For this review, take the finished solid that the model builds, in its own axes (mm). A direction names the side the tool comes from. Round coordinates to 2 decimals unless told otherwise and drop trailing zeros. Write each loop counter-clockwise with the first axis right and the second up, starting at its lowest first coordinate (ties: lowest second). Pieces come first, ordered by that corner, then holes. Notation, with made-up numbers: (75.5, 46) -> (131.5, 46) arc R10 ccw to (131.5, 63) -> close; hole circle Ø7 at (-38.5, 22.5). An arc over 180 degrees is marked (long way). Write each question's results on one line, items separated by ' | '. Start each with the question number.
Item 1: Add section D-D (x = -91). State the section outline as (y, z) points.
Item 2: Add section A-A (y = 0). State the section outline as (x, z) points.
Item 3: Add section C-C (z = 278). State the section outline as (x, y) points, plus the area to 3 significant figures.
Item 4: Tool access review of faces 5 (the flat face through (-1, 111, -45.487)), 6 (the flat face through (2, -54, 0)), 7 (the cylindrical face through (124.88, 5.5, -57.89)): name each direction out of +Z, -Z, +X, -X, +Y, -Y from which nothing blocks a thin tool from reaching the whole face with its end or side.
Item 5: To check wall thickness, follow line 1 along Z through (x, y) = (-100, -70.5); line 2 along Z through (x, y) = (-71, -68.5); line 3 along Y through (x, z) = (32, 986). State the ranges of each line that lie inside material, in increasing order.
Item 6: The part is to be moulded in two halves that separate along Z. For faces 1 (the flat face through (-1, 111, -25.487)), 2 (the flat face through (-1, 1, 1200)), 3 (the cylindrical face through (47.69, 15.02, 591.6)), 4 (the flat face through (2, 2, -70.65)), say which applies: +Z half, -Z half, draft (parallel to the pull), parting line (faces both ways), or undercut.
Item 7: Clearance check with flat-ended pins moving along their axes: pin 1 (5 mm diameter, centred on x = -42, z = 1028, fed in from -Y); pin 2 (6 mm diameter, centred on x = 32, z = 545.5, fed in from +Y); pin 3 (1 mm diameter, centred on y = 17.5, z = 1015.5, fed in from -X). State where each tip first meets the part, or that it passes through.
from build123d import *

# Parameters (mm, degrees)
SKETCH1_R           = 50
BOSS_EXTRUDE1_DEPTH = 1200
SKETCH2_R           = 125
BOSS_EXTRUDE2_DEPTH = 70.65
SKETCH5_W           = 15
SKETCH5_H           = 20


with BuildPart() as part:
    # Sketch1 → Boss-Extrude1 (new body)
    with BuildSketch(Plane.XY):
        Circle(SKETCH1_R)
    extrude(amount=BOSS_EXTRUDE1_DEPTH)

    # Sketch2 → Boss-Extrude2 (add)
    with BuildSketch(Plane(origin=(0, 0, 0), x_dir=(-1, 0, 0), z_dir=(0, 0, -1))):
        Circle(SKETCH2_R)
    extrude(amount=BOSS_EXTRUDE2_DEPTH)

    # Sketch5 → Cut-Revolve1 (revolve, cut)
    with BuildSketch(Plane(origin=(0, 0, 0), x_dir=(1, 0, 0), z_dir=(0, 1, 0)), mode=Mode.PRIVATE) as cut_revolve1_sk:
        with Locations((-117.5, 35.486594565)):
            Rectangle(SKETCH5_W, SKETCH5_H)
    revolve(cut_revolve1_sk.sketch.rotate(Axis((0, 0, 1200), (0, 0, -1)), 180), axis=Axis((0, 0, 1200), (0, 0, -1)), mode=Mode.SUBTRACT)


solid = part.part
Responses:
1) outline: (-85.7, -70.65) -> (85.7, -70.65) -> (85.7, -45.49) -> (61.8, -45.49) -> (61.8, -25.49) -> (85.7, -25.49) -> (85.7, 0) -> (-85.7, 0) -> (-85.7, -25.49) -> (-61.8, -25.49) -> (-61.8, -45.49) -> (-85.7, -45.49) -> close
2) outline: (-125, -70.65) -> (125, -70.65) -> (125, -45.49) -> (110, -45.49) -> (110, -25.49) -> (125, -25.49) -> (125, 0) -> (50, 0) -> (50, 1200) -> (-50, 1200) -> (-50, 0) -> (-125, 0) -> (-125, -25.49) -> (-110, -25.49) -> (-110, -45.49) -> (-125, -45.49) -> close
3) outline: circle Ø100 at (0, 0) | area: 7,850 mm^2
4) face 5: none | face 6: +Z | face 7: +Z, -Z
5) line 1: z = -70.65 to -45.49, -25.49 to 0 | line 2: z = -70.65 to 0 | line 3: y = -38.42 to 38.42
6) face 1: undercut | face 2: +Z half | face 3: draft | face 4: -Z half
7) pin 1: stops at y = -30.66 | pin 2: stops at y = 40.73 | pin 3: stops at x = -47.02
